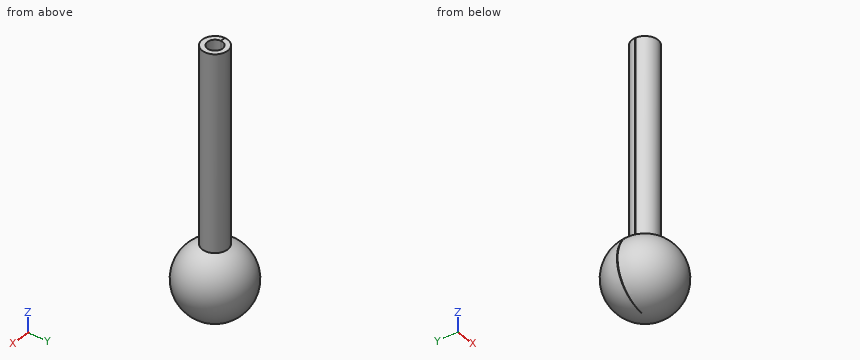
from build123d import *

# Parameters (mm, degrees)
REVOLVE4_ANGLE     = 359
SKETCH9_R          = 6
CUT_EXTRUDE2_DEPTH = 113


with BuildPart() as part:
    # Sketch2 → Revolve4 (revolve)
    with BuildSketch(Plane(origin=(0, 0, 0), x_dir=(1, 0, 0), z_dir=(0, 1, 0))):
        with BuildLine():
            Line((0, 28.377137052), (0, -28.377137052))
            ThreePointArc((0, -28.377137052), (-28.377137052, 0), (0, 28.377137052))
        make_face()
        with BuildLine():
            Line((0, -178.377137052), (0, -28.377137052))
            ThreePointArc((0, -28.377137052), (-5.082168455, -27.91833575), (-10, -26.556767636))
            Line((-10, -26.556767636), (-10, -178.377137052))
            Line((-10, -178.377137052), (0, -178.377137052))
        make_face()
    revolve(axis=Axis((0, 0, 28.377137052), (0, 0, 1)), revolution_arc=REVOLVE4_ANGLE)

    # Sketch9 → Cut-Extrude2 (cut)
    with BuildSketch(Plane.XY.offset(178.377137052)):
        Circle(SKETCH9_R)
    extrude(amount=-CUT_EXTRUDE2_DEPTH, mode=Mode.SUBTRACT)


solid = part.part
Can you work these out from the model? Positions are in its coordinate system, mm. Round coordinates to 2 decimals unless told otherwise and drop trailing zeros. Order: outer loops, then holes, each group sorted by start corner. A loop starts at its lowest first (then second) coordinate and runs counter-clockwise, first axis right, second up. Notation, with made-up numbers: (6.5, 48.5) -> (34.5, 48.5) arc R15 cw to (34.5, 69.5) -> close; hole circle Ø8 at (49, -28.75). An arc over 180 degrees is marked (long way). Write each question's results on one line, items separated by ' | '. Start each with the question number.
Item 1: Will these pins go through, and if not, where does the flat tip stop? pin 1 (8 mm diameter, centred on y = 4, z = 49, fed in from -X); pin 2 (3 mm diameter, centred on x = 15, y = 6.5, fed in from +Z); pin 3 (3 mm diameter, centred on x = 2.5, y = 1.5, fed in from +Z).
Item 2: If we section it at C-C, the plane y = 19: Write out the boundary of the cut face in (x, z), then the cut area to 3 significant figures.
Item 3: Please list where these lines run through material, in increasing order: L1, parallel to Y at x = 4.5, z = 97; L2, parallel to Z at x = 11, y = 22; L3, parallel to X at y = -4, z = 14.
Item 4: If we section it at B-B, the plane z = 121: Write out the boundary of the cut face in (x, y).
Item 5: If we section it at A-A, the plane x = -2.5: Write out the boundary of the cut face in (y, z), then the cut area to 3 significant figures.
Results:
1) pin 1: stops at x = -10 | pin 2: stops at z = 24.18 | pin 3: stops at z = 65.38
2) outline: circle Ø42.16 at (0, 0) | area: 1,400 mm2
3) L1: y = -8.93 to -3.97, 3.97 to 8.93 | L2: z = -14.15 to 14.15 | L3: x = -24.36 to 24.36
4) outline: (-10, 0) arc R10 ccw (long way) to (-10, 0.17) -> (-6, 0.1) arc R6 cw (long way) to (-6, 0) -> close
5) outline: (-9.68, 26.56) arc R28.27 ccw to (0, -28.27) -> (0, 65.38) -> (-5.45, 65.38) -> (-5.45, 178.38) -> (-9.68, 178.38) -> close; (0.04, -28.27) arc R28.27 ccw to (9.68, 26.56) -> (9.68, 178.38) -> (5.45, 178.38) -> (5.45, 65.38) -> (0.04, 65.38) -> close | area: 4,190 mm2
